Work out the finished part from the listing and answer in its coordinate system (mm). Face numbers are marked on the shaded views. A direction names the side the tool comes from. Give positions to 0.01 mm unless a question says otherwise; leave off trailing zeros. Order: outer loops, then holes, each group sorted by start corner. A loop starts at its lowest first (then second) coordinate and runs counter-clockwise, first axis right, second up. Notation, with made-up numbers: M -31.5,-24.5 L -12.5,-24.5 A19 ccw -12.5,11.5 Z; hole C 0.5,45.25 d2. An arc over 180 degrees is marked long. One line per item, written item: value.
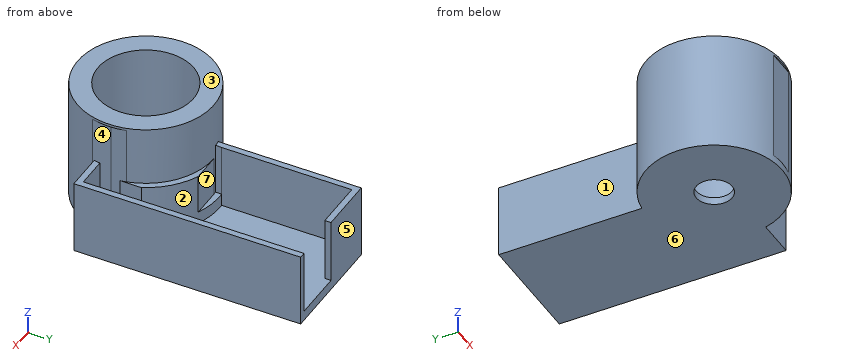
from build123d import *
from build123d.topology import SkipClean

# Parameters (mm, degrees)
BOSS_EXTRUDE1_DEPTH     = 24
CUT_EXTRUDE1_DEPTH      = 91.21363533302491
CUT_EXTRUDE1_DEPTH_BACK = 91.21363533302491
SKETCH2_4_R             = 16.25
CUT_EXTRUDE2_DEPTH      = 3
CUT_EXTRUDE2_DEPTH_BACK = 48
SKETCH2_5_R             = 19.5
SKETCH2_5_R_2           = 16.25
CUT_EXTRUDE3_DEPTH      = 48
CUT_EXTRUDE3_DEPTH_BACK = 16
SKETCH3_W               = 8.5
SKETCH3_H               = 14.200000000000006
CUT_EXTRUDE4_DEPTH      = 40
SKETCH7_R               = 27.499999999999996
SKETCH7_R_2             = 18.9
BOSS_EXTRUDE2_DEPTH     = 1
SKETCH8_W               = 181.3602376825947
SKETCH8_H               = 155.21218123297842
CUT_EXTRUDE5_DEPTH      = 48
BOSS_EXTRUDE3_START     = 48
SKETCH9_R               = 27.499999999999996
SKETCH9_R_2             = 18.9
BOSS_EXTRUDE3_DEPTH     = 48
CUT_EXTRUDE6_DEPTH      = 48
BOSS_EXTRUDE4_DEPTH     = 4
EXTRUDE_THIN2_DEPTH     = 30
CUT_EXTRUDE8_START      = -21
CUT_EXTRUDE8_DEPTH      = 21
BOSS_EXTRUDE5_DEPTH     = 21
CUT_EXTRUDE9_DEPTH      = 21
CUT_EXTRUDE10_DEPTH     = 5
SKETCH21_R              = 27.499999999999996
SKETCH21_R_2            = 7.25
BOSS_EXTRUDE6_DEPTH     = 3
SKETCH24_W              = 354.97877750373505
SKETCH24_H              = 136.88577918663822
CUT_EXTRUDE13_DEPTH     = 109.99999999999999
SKETCH25_R              = 19.3
CUT_EXTRUDE14_DEPTH     = 46


with BuildPart() as part:
    # Sketch2 → Boss-Extrude1 (new, symmetric)
    with BuildSketch(Plane.XY):
        with BuildLine():
            ThreePointArc((-24.69493875270801, -42.900000000000006), (1.68e-15, -82.5), (24.694938752708016, -42.9))
            ThreePointArc((24.694938752708016, -42.9), (21.124860801609124, -27.49999999999999), (24.694938752708012, -12.099999999999996))
            ThreePointArc((24.694938752708012, -12.099999999999996), (3.42e-15, 27.499999999999996), (-24.694938752708012, -12.100000000000001))
            ThreePointArc((-24.694938752708012, -12.100000000000001), (-21.124860801609117, -27.500000000000004), (-24.69493875270801, -42.900000000000006))
        make_face()
    extrude(amount=BOSS_EXTRUDE1_DEPTH, both=True)

    # Sketch2<4> → Cut-Extrude1 (cut, two sides: drawn at the far end of the back side and taken through both)
    with BuildSketch(Plane.XY.offset(-CUT_EXTRUDE1_DEPTH_BACK)):
        with Locations((6.74e-15, -55)):
            Circle(SKETCH2_4_R)
    extrude(amount=CUT_EXTRUDE1_DEPTH + CUT_EXTRUDE1_DEPTH_BACK, mode=Mode.SUBTRACT)

    # Sketch2<5> → Cut-Extrude2 (cut, two sides: drawn at the far end of the back side and taken through both)
    with BuildSketch(Plane.XY.offset(-CUT_EXTRUDE2_DEPTH_BACK)):
        with Locations((6.74e-15, -55)):
            Circle(SKETCH2_5_R)
        with Locations((6.74e-15, -55)):
            Circle(SKETCH2_5_R_2, mode=Mode.SUBTRACT)
    extrude(amount=CUT_EXTRUDE2_DEPTH + CUT_EXTRUDE2_DEPTH_BACK, mode=Mode.SUBTRACT)

    # Sketch2<6> → Cut-Extrude3 (cut, two sides: drawn at the far end of the back side and taken through both)
    with BuildSketch(Plane.XY.offset(-CUT_EXTRUDE3_DEPTH_BACK)):
        Polygon((10.399999999999997, 20.400000000000002), (-10.400000000000002, 20.400000000000002), (-10.399999999999999, -20.399999999999995), (10.400000000000002, -20.399999999999995), align=None)
    extrude(amount=CUT_EXTRUDE3_DEPTH + CUT_EXTRUDE3_DEPTH_BACK, mode=Mode.SUBTRACT)

    # Sketch3 → Cut-Extrude4 (cut)
    with BuildSketch(Plane.XY.offset(24)):
        with Locations((0, 27.500000000000007)):
            Rectangle(SKETCH3_W, SKETCH3_H)
    extrude(amount=-CUT_EXTRUDE4_DEPTH, mode=Mode.SUBTRACT)

    # Sketch7 → Boss-Extrude2 (add)
    with BuildSketch(Plane(origin=(0, 0, -24), x_dir=(-1, 0, 0), z_dir=(0, 0, -1))):
        with Locations((-6.74e-15, -55)):
            Circle(SKETCH7_R)
        with Locations((-6.74e-15, -55)):
            Circle(SKETCH7_R_2, mode=Mode.SUBTRACT)
    extrude(amount=BOSS_EXTRUDE2_DEPTH)

    # Sketch8 → Cut-Extrude5 (cut)
    with BuildSketch(Plane.XY.offset(24)):
        with Locations((-25.06580059332441, -26.494305521168478)):
            Rectangle(SKETCH8_W, SKETCH8_H)
    extrude(amount=-CUT_EXTRUDE5_DEPTH, mode=Mode.SUBTRACT)

    # Sketch9 → Boss-Extrude3 (add)
    with SkipClean():  # the faces are left unmerged after this step: merging them gives an invalid solid
        with BuildSketch(Plane.XY.offset(-24).offset(BOSS_EXTRUDE3_START)):
            with Locations(Location((6.74e-15, -55, 0), (0, 0, 180))):
                Circle(SKETCH9_R)
            with Locations((6.74e-15, -55)):
                Circle(SKETCH9_R_2, mode=Mode.SUBTRACT)
        extrude(amount=-BOSS_EXTRUDE3_DEPTH)

    # Sketch10 → Cut-Extrude6 (cut)
    with SkipClean():  # the faces are left unmerged after this step: merging them gives an invalid solid
        with BuildSketch(Plane.XY.offset(24)):
            with BuildLine():
                Line((26.717930940571712, -48.48830542371335), (26.510281823927063, -55))
                Line((26.510281823927063, -55), (26.510281823927063, -62.311289736835946))
                ThreePointArc((26.51028182392707, -62.311289736835946), (27.25144721072622, -58.68898697761363), (27.500000000000014, -55))
                ThreePointArc((27.500000000000014, -55), (27.30378271289276, -51.72075472598662), (26.717930940571723, -48.48830542371334))
            make_face()
            with BuildLine():
                ThreePointArc((-5.604082705298323, -81.92293180603063), (6e-15, -82.5), (5.604082705298339, -81.92293180603063))
                Line((5.604082705298337, -81.92293180603063), (6.74e-15, -81.92293180603063))
                Line((7.11e-15, -81.92293180603063), (-5.604082705298323, -81.92293180603063))
            make_face()
        extrude(amount=-CUT_EXTRUDE6_DEPTH, mode=Mode.SUBTRACT)

    # Sketch11 → Boss-Extrude4 (add)
    with SkipClean():  # the faces are left unmerged after this step: merging them gives an invalid solid
        with BuildSketch(Plane.XY.offset(24)):
            with BuildLine():
                ThreePointArc((27.500000000000025, -55.00000000000003), (27.300326018506244, -58.3078995273848), (26.7042036884893, -61.56776258429582))
                Line((26.70420368848926, -61.56776258429563), (42.21724684134985, -61.56776258429563))
                Line((42.21724684134985, -61.56776258429563), (42.21724684134985, 29.98869686217629))
                Line((42.21724684134985, 29.988696862176287), (-3.7193423220770256, 29.988696862176287))
                Line((-3.719342322077025, 29.988696862176287), (-3.719342322077025, -27.7526791648939))
                ThreePointArc((-3.719342322077028, -27.7526791648939), (15.483065545848751, -32.27282064789051), (26.717930940571723, -48.488305423713314))
                ThreePointArc((26.717930940571723, -48.488305423713314), (27.303782712892772, -51.72075472598662), (27.500000000000025, -55.00000000000002))
            make_face()
        extrude(amount=-BOSS_EXTRUDE4_DEPTH)

    # Sketch16 → Extrude-Thin2 (add)
    with SkipClean():  # the faces are left unmerged after this step: merging them gives an invalid solid
        with BuildSketch(Plane(origin=(0, 0, 24), x_dir=(-1, 0, 0), z_dir=(0, 0, -1))):
            with BuildLine():
                Line((-26.704203688489347, -61.56776258429563), (-42.21724684134985, -61.56776258429563))
                Line((-42.21724684134985, -61.56776258429563), (-42.21724684134985, 29.988696862176287))
                Line((-42.21724684134985, 29.988696862176287), (3.719342322077025, 29.988696862176287))
                Line((3.719342322077025, 29.988696862176287), (3.719342322077025, -27.75267916489391))
                ThreePointArc((3.719342322077025, -27.75267916489391), (-20.443603637167037, -36.60682000505511), (-26.704203688489347, -61.56776258429563))
            make_face()
            with BuildLine():
                Line((-29.722942444479006, -59.06776258429563), (-39.71724684134985, -59.06776258429563))
                Line((-39.71724684134985, -59.06776258429563), (-39.71724684134985, 27.48869686217629))
                Line((-39.71724684134985, 27.48869686217629), (1.2193423220770256, 27.488696862176287))
                Line((1.2193423220770256, 27.488696862176287), (1.2193423220770252, -25.02479017084956))
                ThreePointArc((1.2193423220770252, -25.02479017084956), (-22.200108055370485, -34.82191281786335), (-29.722942444479006, -59.06776258429563))
            make_face(mode=Mode.SUBTRACT)
        extrude(amount=EXTRUDE_THIN2_DEPTH)

    # Sketch17 → Cut-Extrude8 (cut)
    with BuildSketch(Plane(origin=(0, 0, -5.999999999999998), x_dir=(-1, 0, 0), z_dir=(0, 0, -1)).offset(CUT_EXTRUDE8_START)):
        with BuildLine():
            Line((1.3487027041950868, -27.533092620105528), (1.2193423220770252, -25.02479017084956))
            ThreePointArc((1.2193423220770252, -25.02479017084956), (-22.20010805537015, -34.82191281786366), (-29.72294244447902, -59.06776258429561))
            Line((-29.72294244447902, -59.06776258429561), (-27.19748715520997, -59.06776258429561))
            ThreePointArc((-27.19748715520997, -59.06776258429561), (-20.387465924836167, -36.54461506324914), (1.3487027041950868, -27.533092620105528))
        make_face()
    extrude(amount=CUT_EXTRUDE8_DEPTH, mode=Mode.SUBTRACT)

    # Sketch18 → Boss-Extrude5 (add)
    with BuildSketch(Plane(origin=(0, 0, 20), x_dir=(-1, 0, 0), z_dir=(0, 0, -1))):
        with BuildLine():
            ThreePointArc((-27.19748715520984, -50.93223741570337), (-17.949742740939968, -34.16597169210712), (-1.0275e-13, -27.499999999999904))
            Line((-1.0275e-13, -27.499999999999908), (-11.98957880828152, -27.499999999999908))
            ThreePointArc((-11.98957880828161, -27.49999999999943), (-20.951294804022364, -33.528082385707165), (-27.197487155209934, -42.33916699256241))
            Line((-27.197487155209956, -42.339166992562404), (-27.197487155209956, -50.93223741570336))
        make_face()
    extrude(amount=BOSS_EXTRUDE5_DEPTH)

    # Sketch19 → Cut-Extrude9 (cut)
    with BuildSketch(Plane(origin=(0, 0, -5.999999999999998), x_dir=(-1, 0, 0), z_dir=(0, 0, -1))):
        Polygon((-39.71724684134985, 27.48869686217629), (-39.71724684134984, 29.988696862176287), (-19.248952259636408, 29.988696862176287), (-19.24895225963641, 27.48869686217629), align=None)
    extrude(amount=-CUT_EXTRUDE9_DEPTH, mode=Mode.SUBTRACT)

    # Sketch20 → Cut-Extrude10 (cut)
    with BuildSketch(Plane(origin=(0, 0, 15.000000000000004), x_dir=(-1, 0, 0), z_dir=(0, 0, -1))):
        Polygon((-19.248952259636408, 29.988696862176287), (-39.71724684134984, 29.988696862176287), (-39.71724684134984, 27.48869686217629), (-19.24895225963641, 27.48869686217629), align=None)
    extrude(amount=-CUT_EXTRUDE10_DEPTH, mode=Mode.SUBTRACT)

    # Sketch21 → Boss-Extrude6 (add)
    with BuildSketch(Plane.XY.offset(24)):
        with Locations(Location((6.74e-15, -55, 0), (0, 0, 180))):
            Circle(SKETCH21_R)
        with Locations((6.74e-15, -55)):
            Circle(SKETCH21_R_2, mode=Mode.SUBTRACT)
    extrude(amount=-BOSS_EXTRUDE6_DEPTH)


with BuildPart() as body_2:
    # Mirror1: mirrored copy
    add(part.part.mirror(Plane.XY.offset(34)))

    # Sketch25 → Cut-Extrude14 (cut)
    with BuildSketch(Plane.XY.offset(93)):
        with Locations((6.74e-15, -55)):
            Circle(SKETCH25_R)
    extrude(amount=-CUT_EXTRUDE14_DEPTH, mode=Mode.SUBTRACT)


with BuildPart() as part_1:
    add(part.part)

    # Sketch24 → Cut-Extrude13 (cut)
    with BuildSketch(Plane.XY.offset(24)):
        with Locations((-135.2721419105177, -38.45419273114281)):
            Rectangle(SKETCH24_W, SKETCH24_H)
    extrude(amount=-CUT_EXTRUDE13_DEPTH, mode=Mode.SUBTRACT)


solid = body_2.part
(1) Given P1, Ø1.3, axis at x = 8, y = -26, coming from the +Z side; P2, Ø8, axis at x = 10, y = -16.5, coming from the +Z side; P3, Ø16.5, axis at x = 5, z = 66.5, coming from the -Y side; P4, Ø12, axis at x = 33, y = -66, coming from the -Z side, each flat-ended and moving along its own axis, determine where each tip first touches the part or whether it passes through.
Findings:
P1: stops at z = 53
P2: stops at z = 48
P3: stops at y = -81.92
P4: stops at z = 44
(2) Section B-B, the plane z = 87 is taken. Give the vertices of the cut face in (x, y).
Findings:
outline: M -5.6,-81.92 L 5.6,-81.92 A27.5 ccw 26.51,-62.31 L 26.51,-55 L 26.72,-48.49 A27.5 ccw long Z; hole C 0,-55 d38.6
(3) Section D-D, the plane y = -32.5 is taken. Give the vertices of the cut face in (x, z), then the cut area to 3 significant figures.
Findings:
outline: M -15.81,44 L 42.22,44 L 42.22,74 L 39.72,74 L 39.72,48 L 19.84,48 L 19.84,69 L 15.81,69 L 15.81,93 L -15.81,93 Z
area: 1,800 mm^2
(4) Which of the six approach directions +Z, -Z, +X, -X, +Y, -Y give full straight-line access (tool end or side, diameter ignored) to the marked faces 1, 2, 3 and 4?
Findings:
face 1: +Z, -Z, -X, +Y
face 2: +Z
face 3: +Z, +X, -X, +Y, -Y
face 4: -Y
(5) Determine the mould class of the marked faces 5, 6 and 7 for opening direction Y: pulls with the +Y half, pulls with the -Y half, needs draft (parallel to the pull), parting line crosses it, or undercut.
Findings:
face 5: pulls with the +Y half
face 6: needs draft
face 7: undercut
(6) Find the intervals of material crossed by probe 1 along Y at (x, z) = (1, 64); probe 2 along X at (y, z) = (-8, 51); probe 3 along Y at (x, z) = (0, 45.9), in increasing order. Write a range as from..to.
Findings:
probe 1: y = -81.92..-74.27, -35.73..-27.5, 27.49..29.99
probe 2: x = -3.72..-1.22, 39.72..42.22
probe 3: y = -82.5..-62.25, -47.75..29.99
(7) Section C-C, the plane x = -11 is taken. Give the vertices of the cut face in (y, z), then the cut area to 3 significant figures.
Findings:
outline: M -80.2,44 L -29.8,44 L -29.8,93 L -39.14,93 L -39.14,47 L -70.86,47 L -70.86,93 L -80.2,93 Z
area: 1,010 mm^2
(8) Section A-A, the plane z = 63 is taken. Give the vertices of the cut face in (x, y).
Findings:
outline: M -5.6,-81.92 L 5.6,-81.92 A27.5 ccw 26.51,-62.31 L 26.51,-55 L 26.72,-48.49 A27.5 cw 27.2,-50.93 L 27.2,-42.34 A30 ccw 11.99,-27.5 L 0,-27.5 A27.5 ccw -1.35,-27.53 L -1.22,-25.02 L -1.22,27.49 L 19.25,27.49 L 19.25,29.99 L -3.72,29.99 L -3.72,-27.75 A27.5 ccw Z; M 26.7,-61.57 L 42.22,-61.57 L 42.22,29.99 L 39.72,29.99 L 39.72,-59.07 L 27.2,-59.07 A27.5 cw Z; hole C 0,-55 d38.6
